Source: three-view drawing plus pictorial views. Frame: mm from the lowest corner of the part. A direction names the side the tool comes from. Give positions to 0.01 mm unless a question says otherwise; leave off trailing zeros. Order: outer loops, then holes, each group sorted by start corner. A loop starts at its lowest first (then second) coordinate and runs counter-clockwise, first axis right, second up. Notation, with made-up numbers: M 19,-15 L 25,-15 A21 ccw 25,17 Z; hole C 33.5,24.5 d9. An arc over 180 degrees is marked long. Use CSV: the item, a comma, the result in double quotes. Start each with the question number.
1. Line query: line 1 along Y through (x, z) = (67.5, 107.5); line 2 along Y through (x, z) = (156, 95); line 3 along Z through (x, y) = (139, 26). Output: solid intervals per line, ascending. Write a range as [from, to].
2. Pin query (flat end, axial travel): P1, Ø12, axis at x = 34.5, z = 123.5, coming from the -Y side; P2, Ø1, axis at y = 55.5, z = 76.5, coming from the +X side; P3, Ø5.5, axis at x = 168, y = 133.5, coming from the -Z side; P4, Ø1, axis at x = 44.5, z = 43, coming from the -Y side. Return the tip coordinate at first contact, or that it passes through.
3. Section query A-A, the plane x = 131. Return the cut outline in (y, z) (3 decimals), plus the area to 3 significant figures.
4. Section query D-D, the plane x = 253.5. Return the cut outline in (y, z), plus the area to 3 significant figures.
5. Section query B-B, the plane z = 45.5. Return the cut outline in (x, y), plus the area to 3 significant figures.
6. Section query C-C, the plane y = 47. Return the cut outline in (x, z).
7. Mould query, pull axis X, two halves, no side actions, for the marked faces 4, 5, 6 and 7. Classes: released by +X, released by -X, zero draft, split by the parting line, or undercut.
8. Reachability of the marked faces 1, 2 and 3 from +Z, -Z, +X, -X, +Y, -Y: full face, straight path, thin tool, end or side. Return the list, or none.
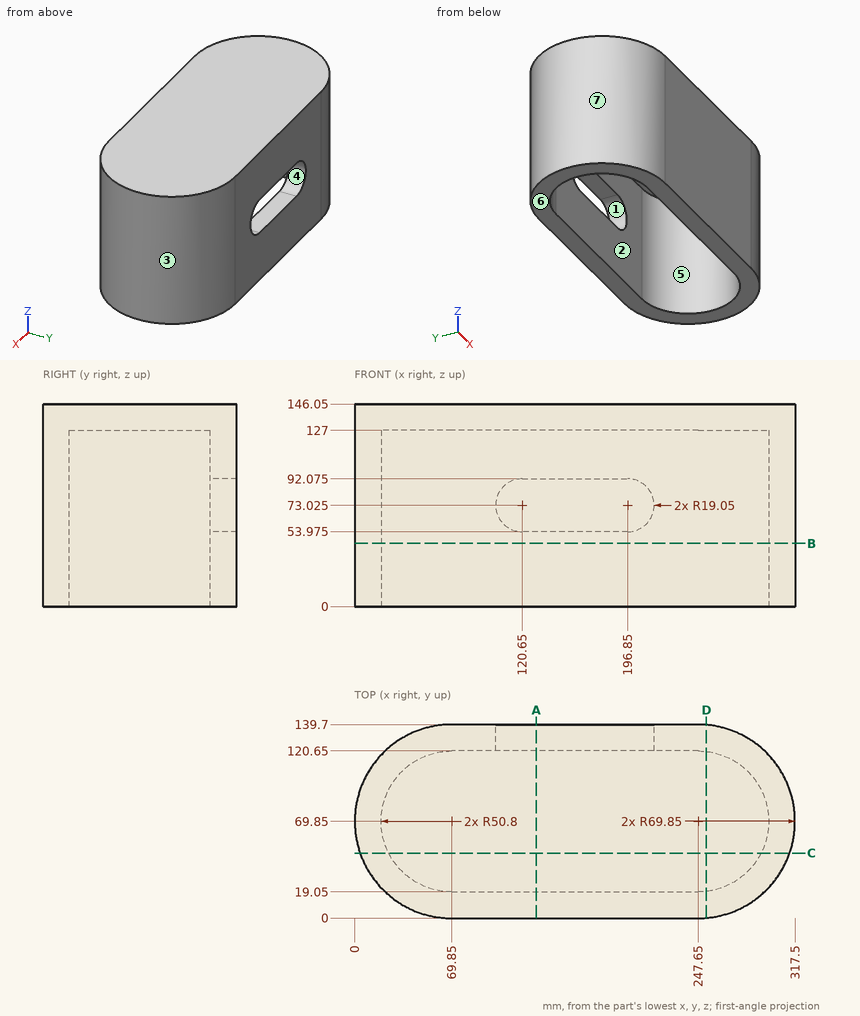
Result set:
1,line 1,"[0.04, 19.1], [120.6, 139.66]"
1,line 2,"[0, 19.05], [120.65, 139.7]"
1,line 3,"[127, 146.05]"
2,P1,"y = 6.47"
2,P2,"x = 316.11"
2,P3,"z = 0"
2,P4,"y = 4.57"
3,outline,"M 0,0 L 19.05,0 L 19.05,127 L 120.65,127 L 120.65,92.075 L 139.7,92.075 L 139.7,146.05 L 0,146.05 Z; M 120.65,0 L 139.7,0 L 139.7,53.975 L 120.65,53.975 Z"
3,area,"6,770 mm2"
4,outline,"M 0.25,0 L 19.39,0 L 19.39,127 L 120.31,127 L 120.31,0 L 139.45,0 L 139.45,146.05 L 0.25,146.05 Z"
4,area,"7,510 mm2"
5,outline,"M 69.85,0 L 247.65,0 A69.85 ccw 247.65,139.7 L 69.85,139.7 A69.85 ccw Z; hole M 69.85,19.05 L 247.65,19.05 A50.8 ccw 247.65,120.65 L 69.85,120.65 A50.8 ccw Z"
5,area,"14,000 mm2"
6,outline,"M 3.84,0 L 24.48,0 L 24.48,127 L 293.02,127 L 293.02,0 L 313.66,0 L 313.66,146.05 L 3.84,146.05 Z"
7,face 4,"undercut"
7,face 5,"undercut"
7,face 6,"zero draft"
7,face 7,"released by -X"
8,face 1,"+Y"
8,face 2,"-Z"
8,face 3,"+Z, -Z, +X"
